Verification items for this drawing (mm, ordinates from the low corner). A direction names the side the tool comes from. Round coordinates to 2 decimals unless told otherwise and drop trailing zeros. Loops run counter-clockwise (first coordinate to the right, second up) from the corner with the lowest first, then second, coordinate; pieces in that order, holes last. Notation, with made-up numbers: (-20.5, 70) -> (34.5, 70) arc R25 cw to (34.5, 83) -> close; hole circle Ø10 at (14, -18.5). An arc over 180 degrees is marked (long way). Use a Markdown table: item, result. Add a question column.
Q1. Set-up check for the marked faces 1, 2 and 3: record each of +Z, -Z, +X, -X, +Y, -Y from which the full face is reachable in a straight line by a thin tool's end or side.
Q2. Sectioned sample at A-A, the plane y = 45.72. Give the number of separate pieces and of enclosed holes in the cut face, then the cut area to 3 significant figures.
Q3. Sectioned sample at C-C, the plane x = 72.39. Enter the section's corners in (y, z) (1 decimal).
Q4. Gauge pin test, flat ends, axial feed: P1, Ø2.5, axis at x = 56.47, y = 20.32, coming from the -Z side; P2, Ø3.5, axis at x = 21.59, y = 57.15, coming from the -Z side; P3, Ø7, axis at x = 56.5, y = 45, coming from the -Z side (3 decimals); P4, Ø3, axis at y = 23, z = 9, coming from the +X side. Record the tip position at first contact, or that the pin passes through.
Q5. Material ranges on L1, parallel to Y at x = 56, z = 10 (1 decimal); L2, parallel to Y at x = 20.32, z = 13.45 (1 decimal); L3, parallel to Y at x = 80.5, z = 6.5, recorded low to high.
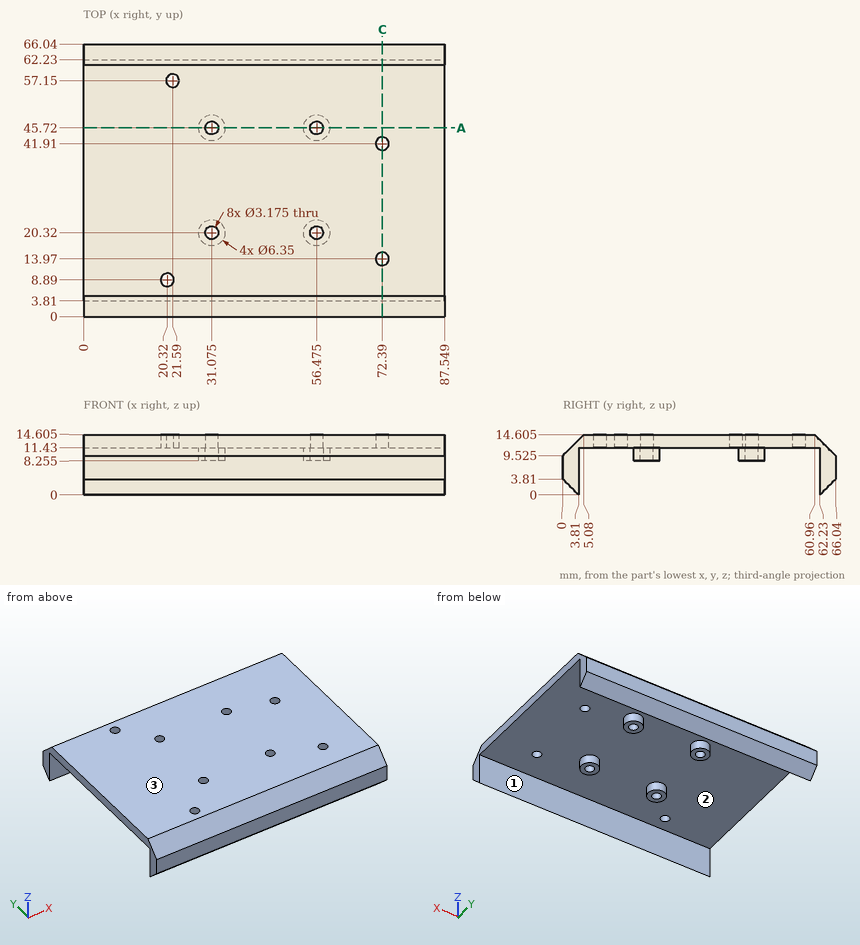
Values:
| question | item | result |
|---|---|---|
| 1 | face 1 | -Z, +X, -X |
| 1 | face 2 | -Z |
| 1 | face 3 | +Z, +X, -X, +Y, -Y |
| 2 | separate pieces | 3 |
| 2 | enclosed holes | 0 |
| 2 | area | 278 mm^2 |
| 3 | outline | (0, 3.8) -> (3.8, 0) -> (3.8, 11.4) -> (12.4, 11.4) -> (12.4, 14.6) -> (5.1, 14.6) -> (0, 9.5) -> close; (15.6, 11.4) -> (40.3, 11.4) -> (40.3, 14.6) -> (15.6, 14.6) -> close; (43.5, 11.4) -> (62.2, 11.4) -> (62.2, 0) -> (66, 3.8) -> (66, 9.5) -> (61, 14.6) -> (43.5, 14.6) -> close |
| 4 | P1 | through |
| 4 | P2 | z = 11.43 |
| 4 | P3 | z = 8.255 |
| 4 | P4 | x = 59.42 |
| 5 | L1 | 0.5 to 3.8, 17.2 to 18.8, 21.8 to 23.5, 42.6 to 44.2, 47.2 to 48.9, 62.2 to 65.6 |
| 5 | L2 | 3.9 to 7.3, 10.5 to 56.2, 58.1 to 62.1 |
| 5 | L3 | 0 to 3.81, 62.23 to 66.04 |
